```python
from build123d import *

# Parameters (mm, degrees)
SKETCH1_W                       = 24
SKETCH1_H                       = 24
SKETCH1_W_2                     = 20
SKETCH1_H_2                     = 20
BOSS_EXTRUDE1_DEPTH             = 20
SKETCH2_W                       = 24
SKETCH2_H                       = 8
SKETCH2_H_2                     = 24
SKETCH2_W_2                     = 20
SKETCH2_H_3                     = 20
BOSS_EXTRUDE2_DEPTH             = 3
F_2_0MM_DOWEL_HOLE1_D           = 2
F_2_0MM_DOWEL_HOLE1_CSINK_D     = 2.05
F_2_0MM_DOWEL_HOLE1_CSINK_ANGLE = 90
F_2_0MM_DOWEL_HOLE2_D           = 2
F_2_0MM_DOWEL_HOLE2_CSINK_D     = 2.05
F_2_0MM_DOWEL_HOLE2_CSINK_ANGLE = 90
FILLET1_R                       = 3
FILLET2_R                       = 2


with BuildPart() as part:
    # Sketch1 → Boss-Extrude1 (new body)
    with BuildSketch(Plane(origin=(0, 0, 0), x_dir=(0, 1, 0), z_dir=(0, 0, 1))):
        Rectangle(SKETCH1_W, SKETCH1_H)
        Rectangle(SKETCH1_W_2, SKETCH1_H_2, mode=Mode.SUBTRACT)
    extrude(amount=BOSS_EXTRUDE1_DEPTH)

    # Sketch2 → Boss-Extrude2 (add)
    # profile 1 of 4: a face of its own
    with BuildSketch(Plane(origin=(0, 0, 0), x_dir=(1, 0, 0), z_dir=(0, 0, -1))):
        with Locations((0, 16)):
            Rectangle(SKETCH2_W, SKETCH2_H)
    # profile 2 of 4: a face of its own
    with BuildSketch(Plane(origin=(0, 0, 0), x_dir=(1, 0, 0), z_dir=(0, 0, -1))):
        with Locations((0, -16)):
            Rectangle(SKETCH2_W, SKETCH2_H)
    # profile 3 of 4: a face of its own
    with BuildSketch(Plane(origin=(0, 0, 0), x_dir=(1, 0, 0), z_dir=(0, 0, -1))):
        Rectangle(SKETCH2_W, SKETCH2_H_2)
        Rectangle(SKETCH2_W_2, SKETCH2_H_3, mode=Mode.SUBTRACT)
    # profile 4 of 4: a face of its own
    with BuildSketch(Plane(origin=(0, 0, 0), x_dir=(1, 0, 0), z_dir=(0, 0, -1))):
        Rectangle(SKETCH2_W_2, SKETCH2_H_3)
    extrude(amount=BOSS_EXTRUDE2_DEPTH)

    # Ø2.0mm Dowel Hole1 (through all)
    with Locations(Plane(origin=(0, 0, -3), x_dir=(1, 0, 0), z_dir=(0, 0, -1))):
        with Locations((7.5, -16), (-27.524465522, 46.822395407), (-7.5, 16), (7.5, 16), (-7.5, -16)):
            CounterSinkHole(F_2_0MM_DOWEL_HOLE1_D / 2, F_2_0MM_DOWEL_HOLE1_CSINK_D / 2, counter_sink_angle=F_2_0MM_DOWEL_HOLE1_CSINK_ANGLE)

    # Ø2.0mm Dowel Hole2 (through all)
    with Locations(Plane(origin=(0, 12, 0), x_dir=(-1, 0, 0), z_dir=(0, 1, 0))):
        with Locations((0, 5)):
            CounterSinkHole(F_2_0MM_DOWEL_HOLE2_D / 2, F_2_0MM_DOWEL_HOLE2_CSINK_D / 2, counter_sink_angle=F_2_0MM_DOWEL_HOLE2_CSINK_ANGLE)

    # Fillet1
    fillet1_edges = [part.edges().sort_by_distance(p)[0] for p in [
        (12, -20, -1.5),
        (-12, -20, -1.5),
        (-12, 20, -1.5),
        (12, 20, -1.5),
    ]]
    fillet(fillet1_edges, radius=FILLET1_R)

    # Fillet2
    fillet2_edges = [part.edges().sort_by_distance(p)[0] for p in [
        (0, 12, 0),
        (0, -12, 0),
    ]]
    fillet(fillet2_edges, radius=FILLET2_R)


solid = part.part
```
Could you check a few things on this model? Use its own coordinates, in mm. A direction names the side the tool comes from. Round coordinates to 2 decimals unless told otherwise and drop trailing zeros. Loops run counter-clockwise (first coordinate to the right, second up) from the corner with the lowest first, then second, coordinate; pieces in that order, holes last. Notation, with made-up numbers: M 87,71.5 L 112,71.5 A16 cw 112,98.5 Z; hole C -39.5,66.25 d3. An arc over 180 degrees is marked long. Write item = value, one per line.
1. I want a section at B-B, the plane x = -7.5. Write out the boundary of the cut face in (y, z) (3 decimals).
Results below:
outline = M -20,-3 L -17.025,-3 L -17,-2.975 L -17,0 L -20,0 Z; M -15,-2.975 L -14.975,-3 L 14.975,-3 L 15,-2.975 L 15,0 L 14,0 A2 cw 12,2 L 12,20 L 10,20 L 10,0 L -10,0 L -10,20 L -12,20 L -12,2 A2 cw -14,0 L -15,0 Z; M 17,-2.975 L 17.025,-3 L 20,-3 L 20,0 L 17,0 Z
2. I want a section at A-A, the plane y = -16. Write out the boundary of the cut face in (x, z) (3 decimals).
Results below:
outline = M -12,-3 L -8.525,-3 L -8.5,-2.975 L -8.5,0 L -12,0 Z; M -6.5,-2.975 L -6.475,-3 L 6.475,-3 L 6.5,-2.975 L 6.5,0 L -6.5,0 Z; M 8.5,-2.975 L 8.525,-3 L 12,-3 L 12,0 L 8.5,0 Z
3. I want a section at C-C, the plane z = 8.5. Write out the boundary of the cut face in (x, y), and give its area (3 significant figures).
Results below:
outline = M -12,-12 L 12,-12 L 12,12 L -12,12 Z; hole M -10,-10 L 10,-10 L 10,10 L -10,10 Z
area = 176 mm²
4. Will these pins go through, and if not, where does the flat tip stop? P1, Ø10, axis at x = 0, y = 3.5, coming from the +Z side; P2, Ø1.6, axis at x = -7.5, y = 16, coming from the +Z side; P3, Ø4, axis at x = 7.5, z = 3.5, coming from the +Y side; P4, Ø5.5, axis at x = 5.5, z = 13.5, coming from the -Y side.
Results below:
P1 = 0
P2 = through
P3 = 12.06
P4 = -12
5. I need wall thicknesses on probe 1 along X at (y, z) = (-16, -1.65); probe 2 along Y at (x, z) = (7.5, -1.15); probe 3 along X at (y, z) = (-9.5, 16). Which ranges of each line are inside material? Lowest first, please.
Results below:
probe_1 = -12 to -8.5, -6.5 to 6.5, 8.5 to 12
probe_2 = -20 to -17, -15 to 15, 17 to 20
probe_3 = -12 to -10, 10 to 12
6. Which directions (+Z, -Z, +X, -X, +Y, -Y) give clear straight access to the entire face, cutting with the end or side of a thin tool? Please do faces 1 (the face through (0, -20, -1)), 2 (the face through (0, 10, 10)), 3 (the face through (0, -17, 0)), 4 (the face through (0, 12, 11)).
Results below:
face_1 = +Z, -Z, +X, -X, -Y
face_2 = +Z
face_3 = +Z, +X, -X, -Y
face_4 = +Z, +X, -X, +Y
7. Thinking about a two-plate mould opening in Y: for faces 5 (the face through (-12, 0, 9)), 6 (the face through (-7.283, 16.976, -1.467)), 7 (the face through (-11.14, 19.1, -1.52)), which applies, +Y half, -Y half, draft (parallel to the pull), parting line (faces both ways), or undercut?
Results below:
face_5 = draft
face_6 = undercut
face_7 = +Y half
8. I want a section at D-D, the plane y = 2. Write out the boundary of the cut face in (x, z), and give its area (3 significant figures).
Results below:
outline = M -12,-3 L 12,-3 L 12,20 L 10,20 L 10,0 L -10,0 L -10,20 L -12,20 Z
area = 152 mm²
